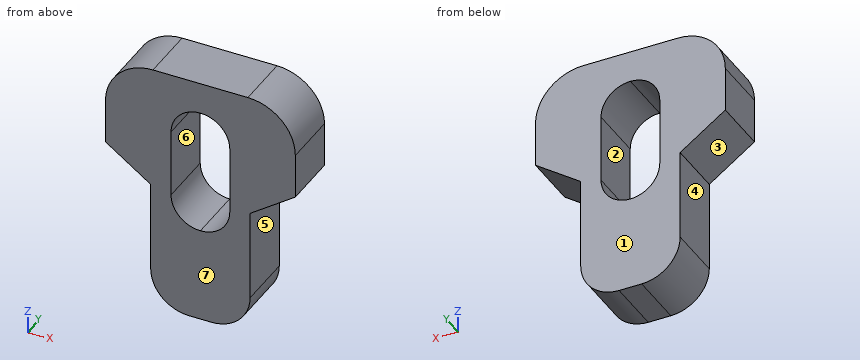
from build123d import *

# Parameters (mm, degrees)
F1_DEPTH = 25


with BuildPart() as f1:
    # F0 (on Front) → F1 (new body)
    with BuildSketch(Plane.XZ):
        with BuildLine():
            Line((-22, 25.36407), (-22, -14.838923))
            ThreePointArc((-22, -14.838923), (-17.020815, -26.859738), (-5, -31.838923))
            Line((-5, -31.838923), (0, -31.838923))
            Line((0, -31.838923), (5, -31.838923))
            ThreePointArc((5, -31.838923), (17.020815, -26.859738), (22, -14.838923))
            Line((22, -14.838923), (22, 25.36407))
            Line((22, 25.36407), (42, 39.36407))
            Line((42, 39.36407), (42, 59.161077))
            ThreePointArc((42, 59.161077), (35.849242, 74.010319), (21, 80.161077))
            Line((21, 80.161077), (0, 80.161077))
            Line((0, 80.161077), (-21, 80.161077))
            ThreePointArc((-21, 80.161077), (-35.849242, 74.010319), (-42, 59.161077))
            Line((-42, 59.161077), (-42, 39.36407))
            Line((-42, 39.36407), (-22, 25.36407))
        make_face()
        with BuildLine():
            ThreePointArc((-13, 53.161077), (-9.192388, 62.353465), (0, 66.161077))
            ThreePointArc((0, 66.161077), (9.192388, 62.353465), (13, 53.161077))
            Line((13, 53.161077), (13, 23.161077))
            ThreePointArc((13, 23.161077), (9.192388, 13.968689), (0, 10.161077))
            ThreePointArc((0, 10.161077), (-9.192388, 13.968689), (-13, 23.161077))
            Line((-13, 23.161077), (-13, 53.161077))
        make_face(mode=Mode.SUBTRACT)
    extrude(amount=F1_DEPTH)


solid = f1.part
Source: CAD feature listing. Evaluate the final solid. Frame: model axes, mm. Face numbers are marked on the shaded views. A direction names the side the tool comes from. Coordinates: 2 decimals unless noted, no trailing zeros. Loops run counter-clockwise (first coordinate to the right, second up) from the corner with the lowest first, then second, coordinate; pieces in that order, holes last. Notation, with made-up numbers: (24.25, 11) - (64.25, 11) arc R24 ccw to (64.25, 22) - close; hole circle Ø5 at (40.5, 83). An arc over 180 degrees is marked (long way). One line per item, written item: value. Start each with the question number.
1. Contact query for flat-ended pins moving along their axis: P1, Ø1.5, axis at x = 23, y = -17, coming from the -Z side; P2, Ø4, axis at x = 29.5, y = -14.5, coming from the +Z side; P3, Ø12.5, axis at y = -12.5, z = -2, coming from the +X side. Output: stop coordinate, or through.
2. Section B-B (z = 62). Return the cut outline in (x, y).
3. Ray query, L1, parallel to X at y = -2.75, z = 46; L2, parallel to X at y = -2, z = 4; L3, parallel to Z at x = 11.5, y = -2.75. Return the intervals inside material, ascending.
4. Section C-C (z = 18.5). Return the cut outline in (x, y), and give its area (3 significant figures).
5. Mould query, pull axis Z, two halves, no side actions, for the marked faces 1, 2 and 3. Classes: pulls with the +Z half, pulls with the -Z half, needs draft (parallel to the pull), parting line crosses it, or undercut.
6. Section A-A (y = -2). Return the cut outline in (x, z).
7. Set-up query: the marked faces 4, 5, 6 and 7. Return all of +Z, -Z, +X, -X, +Y, -Y with unobstructed straight access to the full face (end or side cutting, diameter ignored); none if empty.
8. Section D-D (x = 27). Return the cut outline in (y, z), and give its area (3 significant figures).
Verdict:
1. P1: stops at z = 25.54
1. P2: stops at z = 79.13
1. P3: stops at x = 22
2. outline: (-41.81, -25) - (-9.53, -25) - (-9.53, 0) - (-41.81, 0) - close; (9.53, -25) - (41.81, -25) - (41.81, 0) - (9.53, 0) - close
3. L1: x = -42 to -13, 13 to 42
3. L2: x = -22 to 22
3. L3: z = -30.55 to 17.1, 59.22 to 80.16
4. outline: (-22, -25) - (-12.14, -25) - (-12.14, 0) - (-22, 0) - close; (12.14, -25) - (22, -25) - (22, 0) - (12.14, 0) - close
4. area: 493 mm2
5. face 1: needs draft
5. face 2: undercut
5. face 3: pulls with the -Z half
6. outline: (-42, 39.36) - (-22, 25.36) - (-22, -14.84) arc R17 ccw to (-5, -31.84) - (5, -31.84) arc R17 ccw to (22, -14.84) - (22, 25.36) - (42, 39.36) - (42, 59.16) arc R21 ccw to (21, 80.16) - (-21, 80.16) arc R21 ccw to (-42, 59.16) - close; hole (-13, 23.16) arc R13 ccw to (0, 10.16) arc R13 ccw to (13, 23.16) - (13, 53.16) arc R13 ccw to (0, 66.16) arc R13 ccw to (-13, 53.16) - close
7. face 4: -Z, -X, +Y, -Y
7. face 5: -Z, +X, +Y, -Y
7. face 6: +Y, -Y
7. face 7: +Z, -Z, +X, -X, -Y
8. outline: (-25, 28.86) - (0, 28.86) - (0, 79.29) - (-25, 79.29) - close
8. area: 1,260 mm2
